```python
from build123d import *
from build123d.topology import SkipClean

# Parameters (mm, degrees)
BOSS_EXTRUDE1_START = 24.318234
BOSS_EXTRUDE1_DEPTH = 4
BOSS_EXTRUDE2_DEPTH = 14.010881
REVOLVE1_ANGLE      = 90
BOSS_EXTRUDE3_DEPTH = 114.273182
BOSS_EXTRUDE4_DEPTH = 19.567345
BOSS_EXTRUDE5_DEPTH = 2.39999941


with BuildPart() as part:
    # Sketch4 → Boss-Extrude1 (new body)
    with BuildSketch(Plane.XY.offset(-21.918234102).offset(BOSS_EXTRUDE1_START)):
        Polygon((194.484495585, -141.539185417), (194.484495585, -127.528304219), (314.919807208, -127.528304219), (314.919807208, -25.539185417), (334.487155432, -25.539185417), (334.487155432, -127.528304219), (334.487155432, -141.539185417), align=None)
    extrude(amount=BOSS_EXTRUDE1_DEPTH)

    # Sketch5 → Boss-Extrude2 (add)
    with SkipClean():  # the faces are left unmerged after this step: merging them gives an invalid solid
        with BuildSketch(Plane(origin=(0, -127.528304219, 0), x_dir=(1, 0, 0), z_dir=(0, 1, 0))):
            Polygon((194.484495585, -4.39999941), (188.825701169, 1.263814406), (188.825701169, -6.39999941), (194.484495585, -6.39999941), align=None)
        extrude(amount=-BOSS_EXTRUDE2_DEPTH)

    # Sketch6 → Revolve1 (revolve)
    with BuildSketch(Plane.XZ.offset(141.539185417)):
        Polygon((188.825701169, -1.263814406), (194.484495585, 4.39999941), (194.484495585, 6.39999941), (188.825701169, 6.39999941), align=None)
    revolve(axis=Axis((194.484495585, -141.539185417, 4.39999941), (0, 0, 1)), revolution_arc=REVOLVE1_ANGLE)

    # Sketch7 → Boss-Extrude3 (add)
    with BuildSketch(Plane(origin=(194.484495585, 0, 0), x_dir=(0, 0, -1), z_dir=(1, 0, 0))):
        Polygon((-6.39999941, -147.197979834), (1.263814406, -147.197979834), (-4.39999941, -141.539185417), (-6.39999941, -141.539185417), align=None)
    extrude(amount=BOSS_EXTRUDE3_DEPTH)

    # Sketch9 → Boss-Extrude4 (add)
    with BuildSketch(Plane(origin=(334.487155432, 0, 0), x_dir=(0, 0, -1), z_dir=(1, 0, 0))):
        Polygon((-4.39999941, -25.539185417), (1.201014861, -19.877880744), (-6.39999941, -19.877880744), (-6.39999941, -25.539185417), align=None)
    extrude(amount=-BOSS_EXTRUDE4_DEPTH)


with BuildPart() as boss_extrude5_tool:
    # Sketch11 → Boss-Extrude5 (new body)
    with BuildSketch(Plane(origin=(0, 0, 2.39999941), x_dir=(-1, 0, 0), z_dir=(0, 0, -1))):
        Polygon((-197.504878741, -135.167945919), (-197.504878741, -138.539185417), (-332.752260863, -138.539185417), (-332.932155432, -135.167945919), align=None)
    extrude(amount=BOSS_EXTRUDE5_DEPTH)


with BuildPart() as part_1:
    add(part.part)


with BuildPart() as part_2:
    # Boss-Extrude5: joined with boss_extrude5_tool
    add(part_1.part.fuse(boss_extrude5_tool.part, tol=0.00001))


solid = part_2.part
```
The listing builds one solid part. Answer for the finished solid, in the listing's coordinates (mm). A direction names the side the tool comes from. Coordinates: 2 decimals unless noted, no trailing zeros. Loops run counter-clockwise (first coordinate to the right, second up) from the corner with the lowest first, then second, coordinate; pieces in that order, holes last. Notation, with made-up numbers: (80.5, 77.5) - (92.5, 77.5) arc R23 ccw to (92.5, 97.5) - close; hole circle Ø1 at (-34.5, 43.5). An arc over 180 degrees is marked (long way). Use a Markdown table: item, result. Add a question column.
1) The part is cut by section A-A, the plane x = 225.5. Give the vertices of the cut face in (y, z), and give its area (3 significant figures).
2) The part is cut by section B-B, the plane y = -98.5. Give the vertices of the cut face in (x, z).
3) Given pin 1 (1.2 mm diameter, centred on y = -98.5, z = 3.5, fed in from -X); pin 2 (2.5 mm diameter, centred on x = 251.5, z = 2.5, fed in from +Y); pin 3 (4.5 mm diameter, centred on y = -145.5, z = 0.5, fed in from +X), each flat-ended and moving along its own axis, determine where each tip first touches the part or whether it passes through.
4) For faces 4 (the flat face through (314.92, -77, 4)), 5 (the flat face through (308.758, -145, 3)), 6 (the flat face through (251, -147.198, 3)), determine the directions among +Z, -Z, +X, -X, +Y, -Y from which every point of the face is accessible in a straight line to the end or side of a thin tool.
5) Find the intervals of material crossed by line 1 (Z direction, x = 327, y = -96.5); line 2 (Y direction, x = 300.5, z = 5); line 3 (Y direction, x = 316.5, z = 4.25), in increasing order.
6) The mould has two halves that part along X. Classify faces 1 (the cylindrical face through (190.439, -145.496, 2.514)), 2 (the flat face through (251, -127.528, 4)), 3 (the flat face through (191.695, -134.436, 1.608)): released by +X, released by -X, zero draft, split by the parting line, or undercut.
Here are the results:
| question | item | result |
|---|---|---|
| 1 | outline | (-147.2, -1.26) - (-141.54, 4.4) - (-141.54, 2.4) - (-138.54, 2.4) - (-138.54, 0) - (-135.17, 0) - (-135.17, 2.4) - (-127.53, 2.4) - (-127.53, 6.4) - (-147.2, 6.4) - close |
| 1 | area | 91.5 mm^2 |
| 2 | outline | (314.92, 2.4) - (334.49, 2.4) - (334.49, 6.4) - (314.92, 6.4) - close |
| 3 | pin 1 | stops at x = 314.92 |
| 3 | pin 2 | stops at y = -127.53 |
| 3 | pin 3 | stops at x = 308.76 |
| 4 | face 4 | +Z, -Z, -X, +Y |
| 4 | face 5 | +Z, -Z, +X, -Y |
| 4 | face 6 | +Z, -Z, +X, -X, -Y |
| 5 | line 1 | z = 2.4 to 6.4 |
| 5 | line 2 | y = -147.2 to -127.53 |
| 5 | line 3 | y = -141.54 to -25.54, -25.39 to -19.88 |
| 6 | face 1 | released by -X |
| 6 | face 2 | zero draft |
| 6 | face 3 | undercut |
